```python
from build123d import *

# Parameters (mm, degrees)
LPATTERN1_COUNT       = 11
LPATTERN1_PITCH       = 3
CORTAR_EXTRUIR2_REACH = 35.113
CROQUIS2_R            = 12.499999999999996
CROQUIS2_R_2          = 3.4999999999999982
SKETCH3_R             = 4.8
BOSS_EXTRUDE1_DEPTH   = 3
SKETCH4_R             = 1.75
CUT_EXTRUDE1_DEPTH    = 41.10610926031096
CHAMFER1_SIZE         = 2
SKETCH7_R             = 12.499999999999996
SKETCH7_R_2           = 3.4999999999999982
CUT_EXTRUDE5_DEPTH    = 0.5
CUT_EXTRUDE2_REACH    = 39.437
SKETCH5_R             = 1.2499999999999991
SKETCH5_R_2           = 1.2500000000000002
BOSS_EXTRUDE2_REACH   = 41.211
SKETCH8_R             = 4.999999999999997
SKETCH8_R_2           = 3.4999999999999982
CORTAR_EXTRUIR1_REACH = 39.437
CROQUIS1_R            = 1.5500000000000003


with BuildPart() as part:
    # Sketch1 → Revolve1 (revolve)
    with BuildSketch(Plane.XY, mode=Mode.PRIVATE) as revolve1_sk:
        Polygon((-2.5, -3.1e-16), (-2.5, 5.999999999999998), (-0.7999999999999999, 5.999999999999998), (-0.8, 33), (-12.5, 33), (-12.499999999999995, 0), align=None)
    revolve(revolve1_sk.sketch.rotate(Axis((0, 0, 0), (0, 1, 0)), 270), axis=Axis((0, 0, 0), (0, 1, 0)))

    # Sketch2 → Cut-Revolve1 (revolve, cut)
    with BuildSketch(Plane(origin=(0, 0, 0), x_dir=(0, 0, -1), z_dir=(1, 0, 0))):
        Polygon((12.499999999999996, 30), (3.4999999999999973, 30), (3.499999999999998, 27.999999999999996), (12.499999999999996, 27.999999999999993), align=None)
    cut_revolve1 = revolve(axis=Axis((0, 33, 0), (0, -1, 0)), mode=Mode.SUBTRACT)

    # LPattern1: Cut-Revolve1 ×11
    with Locations(*[(0, -i * LPATTERN1_PITCH, 0) for i in range(1, LPATTERN1_COUNT)]):
        add(cut_revolve1, mode=Mode.SUBTRACT)

    # Croquis2 → Cortar-Extruir2 (cut, up to next)
    with BuildSketch(Plane(origin=(0, 27.999999999999996, 0), x_dir=(1, 0, 0), z_dir=(0, 1, 0)), mode=Mode.PRIVATE) as cortar_extruir2_sk1:
        with Locations(Location((0, 0, 0), (0, 0, 270))):
            Circle(CROQUIS2_R)
        with Locations(Location((0, 0, 0), (0, 0, 270))):
            Circle(CROQUIS2_R_2, mode=Mode.SUBTRACT)
    cortar_extruir2_tool1 = extrude(cortar_extruir2_sk1.sketch, amount=-CORTAR_EXTRUIR2_REACH, mode=Mode.PRIVATE) & part.part
    add(cortar_extruir2_tool1.solids().sort_by_distance((0, 28, -12.146447))[0], mode=Mode.SUBTRACT)

    # Sketch3 → Boss-Extrude1 (add)
    with BuildSketch(Plane(origin=(0, 33, 0), x_dir=(1, 0, 0), z_dir=(0, 1, 0))):
        with Locations(Location((0, 0, 0), (0, 0, 90))):
            Circle(SKETCH3_R)
    extrude(amount=BOSS_EXTRUDE1_DEPTH)

    # Sketch4 → Cut-Extrude1 (cut, through all)
    with BuildSketch(Plane(origin=(0, 36.00000000000001, 0), x_dir=(1, 0, 0), z_dir=(0, 1, 0))):
        with Locations(Location((0, 0, 0), (0, 0, 270))):
            Circle(SKETCH4_R)
    extrude(amount=-CUT_EXTRUDE1_DEPTH, mode=Mode.SUBTRACT)

    # Chamfer1
    chamfer1_edges = [part.edges().sort_by_distance(p)[0] for p in [
        (5.4e-16, 36.00000000000001, -1.75),
    ]]
    chamfer(chamfer1_edges, length=CHAMFER1_SIZE)

    # Sketch7 → Cut-Extrude5 (cut)
    with BuildSketch(Plane(origin=(0, 30, 0), x_dir=(1, 0, 0), z_dir=(0, 1, 0))):
        with Locations(Location((0, 0, 0), (0, 0, 270))):
            Circle(SKETCH7_R)
        with Locations(Location((0, 0, 0), (0, 0, 270))):
            Circle(SKETCH7_R_2, mode=Mode.SUBTRACT)
    extrude(amount=CUT_EXTRUDE5_DEPTH, mode=Mode.SUBTRACT)

    # Sketch5 → Cut-Extrude2 (cut, up to next)
    with BuildSketch(Plane(origin=(0, 33, 0), x_dir=(1, 0, 0), z_dir=(0, 1, 0)), mode=Mode.PRIVATE) as cut_extrude2_sk1:
        with Locations(Location((9, -9.8e-16, 0), (0, 0, 270))):
            Circle(SKETCH5_R)
    cut_extrude2_tool1 = extrude(cut_extrude2_sk1.sketch, amount=-CUT_EXTRUDE2_REACH, mode=Mode.PRIVATE) & part.part
    # Sketch5 → Cut-Extrude2 (cut, up to next)
    with BuildSketch(Plane(origin=(0, 33, 0), x_dir=(1, 0, 0), z_dir=(0, 1, 0)), mode=Mode.PRIVATE) as cut_extrude2_sk2:
        with Locations(Location((-4.499999999999999, -7.794228634059948, 0), (0, 0, 270))):
            Circle(SKETCH5_R_2)
    cut_extrude2_tool2 = extrude(cut_extrude2_sk2.sketch, amount=-CUT_EXTRUDE2_REACH, mode=Mode.PRIVATE) & part.part
    # Sketch5 → Cut-Extrude2 (cut, up to next)
    with BuildSketch(Plane(origin=(0, 33, 0), x_dir=(1, 0, 0), z_dir=(0, 1, 0)), mode=Mode.PRIVATE) as cut_extrude2_sk3:
        with Locations(Location((-4.5000000000000036, 7.794228634059946, 0), (0, 0, 270))):
            Circle(SKETCH5_R_2)
    cut_extrude2_tool3 = extrude(cut_extrude2_sk3.sketch, amount=-CUT_EXTRUDE2_REACH, mode=Mode.PRIVATE) & part.part
    add(cut_extrude2_tool1.solids().sort_by_distance((9, 33, 0))[0], mode=Mode.SUBTRACT)
    add(cut_extrude2_tool2.solids().sort_by_distance((-4.5, 33, 7.794229))[0], mode=Mode.SUBTRACT)
    add(cut_extrude2_tool3.solids().sort_by_distance((-4.5, 33, -7.794229))[0], mode=Mode.SUBTRACT)

    # Boss-Extrude2: up to this face of the body (flat: up to its plane)
    boss_extrude2_end = Plane(part.part.faces().sort_by_distance((0, 9, 12.146446609))[0])
    # Sketch8 → Boss-Extrude2 (add, up to the picked face)
    with BuildSketch(Plane(origin=(0, 0.9999999999999974, 0), x_dir=(1, 0, 0), z_dir=(0, 1, 0)), mode=Mode.PRIVATE) as boss_extrude2_sk1:
        with Locations(Location((0, 0, 0), (0, 0, 90))):
            Circle(SKETCH8_R)
        with Locations(Location((0, 0, 0), (0, 0, 270))):
            Circle(SKETCH8_R_2, mode=Mode.SUBTRACT)
    boss_extrude2_tool1 = split(extrude(boss_extrude2_sk1.sketch, amount=BOSS_EXTRUDE2_REACH, mode=Mode.PRIVATE), bisect_by=boss_extrude2_end, keep=Keep.BOTH, mode=Mode.PRIVATE)
    add(boss_extrude2_tool1.solids().sort_by(Axis((0, 1, 4.858579), (0, 1, 0)))[0])

    # Croquis1 → Cortar-Extruir1 (cut, up to next)
    with BuildSketch(Plane(origin=(0, 33, 0), x_dir=(1, 0, 0), z_dir=(0, 1, 0)), mode=Mode.PRIVATE) as cortar_extruir1_sk1:
        with Locations(Location((4.49999999999998, 7.7942286340599605, 0), (0, 0, 270))):
            Circle(CROQUIS1_R)
    cortar_extruir1_tool1 = extrude(cortar_extruir1_sk1.sketch, amount=-CORTAR_EXTRUIR1_REACH, mode=Mode.PRIVATE) & part.part
    add(cortar_extruir1_tool1.solids().sort_by_distance((4.5, 33, -7.794229))[0], mode=Mode.SUBTRACT)


solid = part.part
```
Part model, mm, in its own coordinate system. A direction names the side the tool comes from. Give positions to 0.01 mm unless a question says otherwise; leave off trailing zeros. Write each loop counter-clockwise with the first axis right and the second up, starting at its lowest first coordinate (ties: lowest second). Pieces come first, ordered by that corner, then holes. Notation, with made-up numbers: (13.5, 14.5) -> (56.5, 14.5) arc R12 cw to (56.5, 28.5) -> close; hole circle Ø1 at (20.25, 16). An arc over 180 degrees is marked (long way). Put each result on its own line as item: value. Start each with the question number.
Item 1: Wall check: L1, parallel to X at y = 32.1, z = 0; L2, parallel to X at y = 19.5, z = 0; L3, parallel to Z at x = 4.5, y = 31.4. Give the ranges that are in metal, low to high. Write a range as [from, to].
Item 2: Pull direction Y, two halves, no side cores. Call faces 1 (the face through (3, 2, 4)), 2 (the face through (-4.98, 31.77, -6.64)): pulls with the +Y half, pulls with the -Y half, needs draft (parallel to the pull), parting line crosses it, or undercut.
Item 3: Cut at B-B (y = 18.5). List the corners of the cut face in (x, z).
Item 4: Cut at A-A (y = 32.5). List the corners of the cut face in (x, z).
Item 5: Cut at C-C (x = 9). State how many separate pieces and enclosed holes the cut face has, then the cut area to 3 significant figures.
Item 6: Pin check, flat tips, straight feed: pin 1 Ø4 at (x, z) = (9, 6) entering from +Y; pin 2 Ø8 at (x, y) = (4, 24.5) entering from +Z; pin 3 Ø4.5 at (x, z) = (0, 0) entering from +Y; pin 4 Ø4 at (y, z) = (14.5, 5.5) entering from +X. Stop position of each tip, or through.
Item 7: Which spindle directions (+Z, -Z, +X, -X, +Y, -Y) get a long thin tool onto all of the face, cutting with end or side? Do faces 3 (the face through (-3.755, 12.493, -11.923)), 4 (the face through (-3, 18, -3)), 5 (the face through (10.24, 31.77, -0.16)). Say none if no direction does.
Answer list:
1. L1: x = [-12.5, -1.75], [1.75, 7.75], [10.25, 12.5]
1. L2: x = [-3.5, -1.75], [1.75, 3.5]
1. L3: z = [-11.66, -9.34], [-6.24, 11.66]
2. face 1: undercut
2. face 2: needs draft
3. outline: circle Ø25 at (0, 0); hole circle Ø3.5 at (0, 0)
4. outline: circle Ø25 at (0, 0); hole circle Ø2.5 at (-4.5, -7.79); hole circle Ø2.5 at (-4.5, 7.79); hole circle Ø3.5 at (0, 0); hole circle Ø3.1 at (4.5, -7.79); hole circle Ø2.5 at (9, 0)
5. separate pieces: 11
5. enclosed holes: 0
5. area: 193 mm2
6. pin 1: stops at y = 33
6. pin 2: stops at z = 12.5
6. pin 3: stops at y = 34.5
6. pin 4: stops at x = 11.98
7. face 3: +Y, -Y
7. face 4: none
7. face 5: +Y
